```python
from build123d import *

# Parameters (mm, degrees)
PAD_DEPTH            = 90
SKETCH004_W          = 5
SKETCH004_H          = 29.8
PAD001_DEPTH         = 4.5
SKETCH001_R          = 2
POCKET_DEPTH         = 4.501
SKETCH005_W          = 1.1
SKETCH005_H          = 40
POCKET001_DEPTH      = 4.501
SKETCH006_R          = 1.5
POCKET002_DEPTH      = 1.951
POCKET002_DEPTH_BACK = -3.051
SKETCH007_R          = 2
POCKET003_DEPTH      = 5


with BuildPart() as part:
    # Sketch → Pad (new body)
    with BuildSketch(Plane.XZ):
        with BuildLine():
            Line((-1.5, 0), (1.5, 0))
            ThreePointArc((1.5, 0), (0, 4.5), (-1.5, 0))
        make_face()
    extrude(amount=PAD_DEPTH)

    # Sketch004 → Pad001 (new body)
    with BuildSketch(Plane(origin=(0, 0, 0), x_dir=(1, 0, 0), z_dir=(0, 0, -1))):
        with Locations((0, 19.9)):
            Rectangle(SKETCH004_W, SKETCH004_H)
    extrude(amount=-PAD001_DEPTH)

    # Sketch001 → Pocket (cut, through all)
    with BuildSketch(Plane(origin=(0, 0, 0), x_dir=(1, 0, 0), z_dir=(0, 0, -1))):
        with Locations((0, 19.9)):
            Circle(SKETCH001_R)
    extrude(amount=-POCKET_DEPTH, mode=Mode.SUBTRACT)

    # Sketch005 → Pocket001 (cut, through all)
    with BuildSketch(Plane(origin=(0, 0, 0), x_dir=(1, 0, 0), z_dir=(0, 0, -1))):
        with Locations((0, 70)):
            Rectangle(SKETCH005_W, SKETCH005_H)
    extrude(amount=-POCKET001_DEPTH, mode=Mode.SUBTRACT)

    # Sketch006 → Pocket002 (cut, two sides)
    with BuildSketch(Plane(origin=(-0.55, 0, 0), x_dir=(0, 0, 1), z_dir=(1, 0, 0))) as pocket002_sk:
        with Locations((2, 60)):
            Circle(SKETCH006_R)
        with Locations((2, 85)):
            Circle(SKETCH006_R)
    extrude(amount=-POCKET002_DEPTH, mode=Mode.SUBTRACT)
    extrude(pocket002_sk.sketch, amount=-POCKET002_DEPTH_BACK, mode=Mode.SUBTRACT)

    # Sketch007 → Pocket003 (cut)
    with BuildSketch(Plane(origin=(0, 0, 0), x_dir=(1, 0, 0), z_dir=(0, 1, 0))):
        with Locations((0, -2)):
            Circle(SKETCH007_R)
    extrude(amount=-POCKET003_DEPTH, mode=Mode.SUBTRACT)


solid = part.part
```
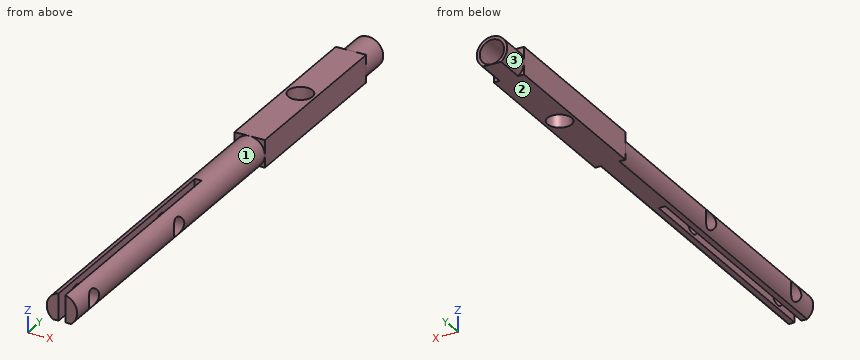
Design review of the part built by this model. Coordinates are the model's own, in mm. Face numbers are marked on the shaded views. A direction names the side the tool comes from. Round coordinates to 2 decimals unless told otherwise and drop trailing zeros. Write each loop counter-clockwise with the first axis right and the second up, starting at its lowest first coordinate (ties: lowest second). Pieces come first, ordered by that corner, then holes. Notation, with made-up numbers: (-2.75, 49) -> (19.25, 49) arc R22 ccw to (19.25, 70) -> close; hole circle Ø3 at (14.5, -27.5). An arc over 180 degrees is marked (long way). Write item = value, one per line. Start each with the question number.
1) Wall thickness on probe 1 along Y at (x, z) = (-0.1, 2.85); probe 2 along Y at (x, z) = (1.15, 1.1); probe 3 along Y at (x, z) = (-1.15, 1.95): over which ranges is each line inside the solid? List them lowest first. Write a range as from..to.
2) Take a section at A-A, the plane y = -19.9. State the section outline as (x, z) points, plus the area to 3 significant figures.
3) Take a section at B-B, the plane y = -85. State the section outline as (x, z) points.
4) Take a section at D-D, the plane y = -72.5. State the section outline as (x, z) points.
5) Tool access review of the marked faces 1, 2 and 3: name each direction out of +Z, -Z, +X, -X, +Y, -Y from which nothing blocks a thin tool from reaching the whole face with its end or side.
6) Take a section at C-C, the plane z = 1.2. Count the separate pieces of the cut face and the enclosed holes in it, plus the area to 3 significant figures.
7) Clearance check with a flat-ended pin moving along its axis: pin 1 (2.5 mm diameter, centred on y = -60, z = 2, fed in from +X). State where the tip first meets the part, or that it passes through.
Results list:
q1.probe_1 = -50..-21.9, -17.9..-5
q1.probe_2 = -90..-86.2, -83.8..-61.2, -58.8..-21.54, -18.26..-5
q1.probe_3 = -90..-86.5, -83.5..-61.5, -58.5..-21.54, -18.26..-5
q2.outline = (-2.5, 0) -> (-2, 0) -> (-2, 4.5) -> (-2.5, 4.5) -> close; (2, 0) -> (2.5, 0) -> (2.5, 4.5) -> (2, 4.5) -> close
q2.area = 4.50 mm²
q3.outline = (-2, 0.5) arc R2.5 ccw to (-1.5, 0) -> (-0.55, 0) -> (-0.55, 0.5) -> close; (-2, 3.5) -> (-0.55, 3.5) -> (-0.55, 4.44) arc R2.5 ccw to start; (0.55, 0) -> (1.5, 0) arc R2.5 ccw to (2, 0.5) -> (0.55, 0.5) -> close; (0.55, 3.5) -> (2, 3.5) arc R2.5 ccw to (0.55, 4.44) -> close
q4.outline = (-1.5, 0) -> (-0.55, 0) -> (-0.55, 4.44) arc R2.5 ccw to start; (0.55, 0) -> (1.5, 0) arc R2.5 ccw to (0.55, 4.44) -> close
q5.face_1 = -Y
q5.face_2 = -Z, +X, -X, +Y, -Y
q5.face_3 = +Y
q6.separate_pieces = 5
q6.enclosed_holes = 1
q6.area = 341 mm²
q7.pin_1 = through
